Can you work these out from the model? Positions are in its coordinate system, mm. Face numbers are marked on the shaded views. A direction names the side the tool comes from. Round coordinates to 2 decimals unless told otherwise and drop trailing zeros. Loops run counter-clockwise (first coordinate to the right, second up) from the corner with the lowest first, then second, coordinate; pieces in that order, holes last. Notation, with made-up numbers: (5.5, -28.75) -> (57.5, -28.75) arc R26 ccw to (57.5, 9.25) -> close; hole circle Ø8 at (52, -2.75). An arc over 180 degrees is marked (long way). Write each question's results on one line, items separated by ' | '.
from build123d import *

# Parameters (mm, degrees)
SKETCH1_W           = 50
SKETCH1_H           = 50
SKETCH1_R           = 3.25
SKETCH1_W_2         = 20
BOSS_EXTRUDE1_DEPTH = 5.3
SKETCH2_R           = 4
BOSS_EXTRUDE2_DEPTH = 50
FILLET1_R           = 3


with BuildPart() as part:
    # Sketch1 → Boss-Extrude1 (new body)
    # profile 1 of 2: a face of its own
    with BuildSketch(Plane(origin=(0, 0, 0), x_dir=(1, 0, 0), z_dir=(0, 1, 0))):
        with Locations((25, -25)):
            Rectangle(SKETCH1_W, SKETCH1_H)
        with Locations(Location((10, -40, 0), (0, 0, 270))):
            Circle(SKETCH1_R, mode=Mode.SUBTRACT)
        with Locations(Location((40, -40, 0), (0, 0, 270))):
            Circle(SKETCH1_R, mode=Mode.SUBTRACT)
        with Locations(Location((40, -10, 0), (0, 0, 270))):
            Circle(SKETCH1_R, mode=Mode.SUBTRACT)
        with Locations(Location((10, -10, 0), (0, 0, 270))):
            Circle(SKETCH1_R, mode=Mode.SUBTRACT)
    # profile 2 of 2: a face of its own
    with BuildSketch(Plane(origin=(0, 0, 0), x_dir=(1, 0, 0), z_dir=(0, 1, 0))):
        with Locations((60, -25)):
            Rectangle(SKETCH1_W_2, SKETCH1_H)
    extrude(amount=BOSS_EXTRUDE1_DEPTH)

    # Sketch2 → Boss-Extrude2 (add)
    with BuildSketch(Plane.XY.offset(50)):
        with BuildLine():
            Line((55, 18.071423244), (55, 5.3))
            Line((55, 5.3), (70, 5.3))
            Line((70, 5.3), (70, 18.071423244))
            ThreePointArc((70, 18.071423244), (62.5, 25.571423244), (55, 18.071423244))
        make_face()
        with Locations((62.5, 18.071423244)):
            Circle(SKETCH2_R, mode=Mode.SUBTRACT)
    extrude(amount=-BOSS_EXTRUDE2_DEPTH)

    # Fillet1
    fillet1_edges = [part.edges().sort_by_distance(p)[0] for p in [
        (55, 5.3, 25),
    ]]
    fillet(fillet1_edges, radius=FILLET1_R)


solid = part.part
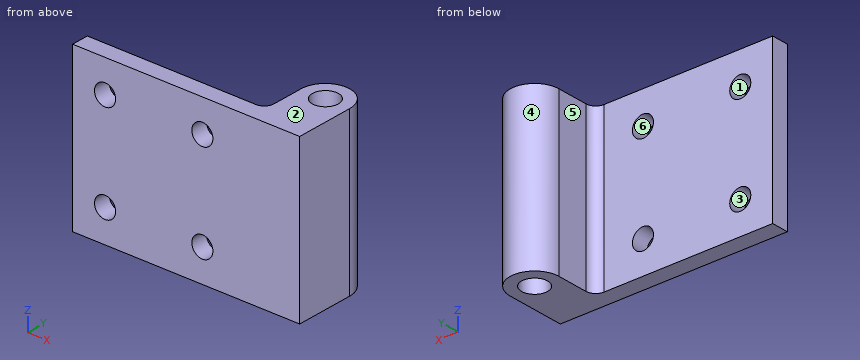
1. Will these pins go through, and if not, where does the flat tip stop? pin 1 (12 mm diameter, centred on y = 18, z = 18, fed in from -X); pin 2 (1 mm diameter, centred on y = 7.5, z = 39.5, fed in from -X); pin 3 (4 mm diameter, centred on x = 62, z = 19.5, fed in from -Y); pin 4 (7.5 mm diameter, centred on x = 10, z = 40, fed in from +Y).
Final values:
pin 1: x = 55 | pin 2: x = 54.7 | pin 3: y = 0 | pin 4: y = 5.3
2. Please list where these lines run through material, in increasing order: line 1 (X direction, y = 2.85, z = 40); line 2 (Y direction, x = 8, z = 48.5); line 3 (X direction, y = 10.5, z = 22). Write a range as from..to.
Final values:
line 1: 0..6.75, 13.25..36.75, 43.25..70 | line 2: 0..5.3 | line 3: 55..70
3. If we section it at A-A (x = 62.5): List the corners of the cut face in (y, z) for me.
Final values:
outline: (0, 0) -> (14.07, 0) -> (14.07, 50) -> (0, 50) -> close; (22.07, 0) -> (25.57, 0) -> (25.57, 50) -> (22.07, 50) -> close
4. If we section it at B-B (z = 10): List the corners of the cut face in (x, y) for me, then the cut area to 3 significant figures.
Final values:
outline: (0, 0) -> (6.75, 0) -> (6.75, 5.3) -> (0, 5.3) -> close; (13.25, 0) -> (36.75, 0) -> (36.75, 5.3) -> (13.25, 5.3) -> close; (43.25, 0) -> (70, 0) -> (70, 18.07) arc R7.5 ccw to (55, 18.07) -> (55, 8.3) arc R3 cw to (52, 5.3) -> (43.25, 5.3) -> close; hole circle Ø8 at (62.5, 18.07) | area: 534 mm2
5. We'd pull the mould along Z, two halves only. Please class the marked faces 1, 2, 3 and 4: pulls with the +Z half, pulls with the -Z half, needs draft (parallel to the pull), parting line crosses it, or undercut.
Final values:
face 1: undercut | face 2: pulls with the +Z half | face 3: undercut | face 4: needs draft
6. If we section it at C-C (x = 40): List the corners of the cut face in (y, z) for me, then the cut area to 3 significant figures.
Final values:
outline: (0, 0) -> (5.3, 0) -> (5.3, 6.75) -> (0, 6.75) -> close; (0, 13.25) -> (5.3, 13.25) -> (5.3, 36.75) -> (0, 36.75) -> close; (0, 43.25) -> (5.3, 43.25) -> (5.3, 50) -> (0, 50) -> close | area: 196 mm2
7. On a 3-axis mill with a long thin cutter (end or side, diameter ignored), from which of +Z, -Z, +X, -X, +Y, -Y can I reach the whole of each face in a straight line? I mean the marked faces 5 and 6. Say none if no direction works.
Final values:
face 5: +Z, -Z, -X, +Y | face 6: +Y, -Y
8. If we section it at D-D (y = 16): List the corners of the cut face in (x, z) for me, then the cut area to 3 significant figures.
Final values:
outline: (55, 0) -> (59.08, 0) -> (59.08, 50) -> (55, 50) -> close; (65.92, 0) -> (70, 0) -> (70, 50) -> (65.92, 50) -> close | area: 408 mm2
